The drawing under review shows one solid part. Ordinate dimensions are in mm from its lowest x, y, z. A direction names the side the tool comes from. Coordinates: 2 decimals unless noted, no trailing zeros. Write each loop counter-clockwise with the first axis right and the second up, starting at its lowest first coordinate (ties: lowest second). Pieces come first, ordered by that corner, then holes.
1) Add section B-B, the plane x = 19.25. State the section outline as (y, z) points, then the cut area to 3 significant figures.
2) Mouldability with a two-part tool opening along X and no side actions: class the marked faces 4, 5 and 6 as released by +X, released by -X, zero draft, split by the parting line, or undercut.
3) For line 1 (X direction, y = 27.5, z = 17.5); line 2 (X direction, y = 28, z = 25.5); line 3 (X direction, y = 15.5, z = 16), list the stretches that pass through material, from the lowest coordinate up.
4) Machinability: for the marked faces 1, 2 and 3, which of the approach directions +Z, -Z, +X, -X, +Y, -Y give a long, thin tool a straight path to every point of the face, cutting with its end or side? Answer none if there is none.
5) Add section C-C, the plane x = 11. State the section outline as (y, z) points.
6) For P1, Ø1, axis at x = 16.5, z = 29.5, coming from the +Y side; P2, Ø5, axis at y = 29, z = 10.5, coming from the +X side; P3, Ø10, axis at y = 18, z = 36, coming from the +X side, all flat-tipped, find the tip position at first contact; note any pin that passes through.
7) Add section A-A, the plane z = 21. State the section outline as (x, y) points.
8) Add section D-D, the plane y = 30. State the section outline as (x, z) points.
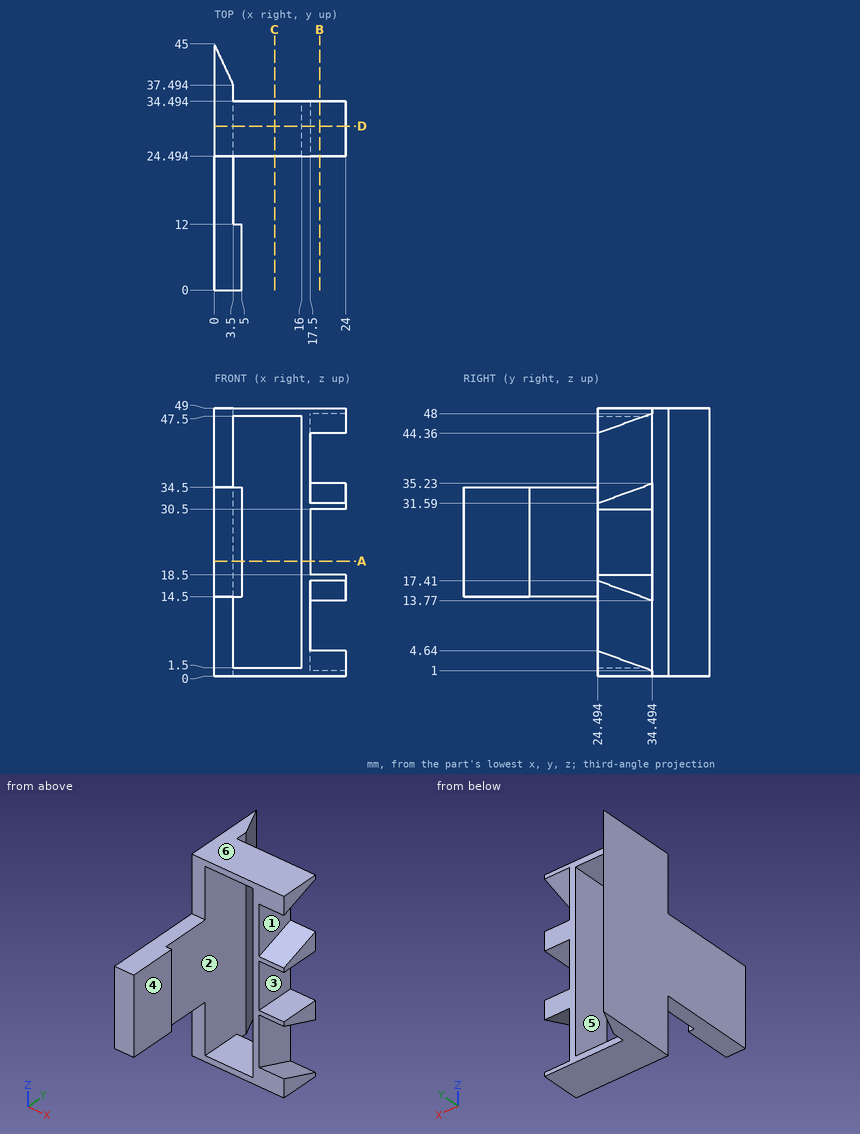
Geometry results:
1. outline: (24.49, 0) - (34.49, 0) - (34.49, 1) - (24.49, 4.64) - close; (24.49, 17.41) - (34.49, 13.77) - (34.49, 18.5) - (24.49, 18.5) - close; (24.49, 30.5) - (34.49, 30.5) - (34.49, 35.23) - (24.49, 31.59) - close; (24.49, 44.36) - (34.49, 48) - (34.49, 49) - (24.49, 49) - close
1. area: 115 mm2
2. face 4: released by +X
2. face 5: undercut
2. face 6: zero draft
3. line 1: x = 0 to 3.5, 16 to 24
3. line 2: x = 0 to 3.5, 16 to 17.5
3. line 3: x = 0 to 3.5
4. face 1: +X
4. face 2: +Y
4. face 3: +X, +Y, -Y
5. outline: (24.49, 0) - (34.49, 0) - (34.49, 1.5) - (24.49, 1.5) - close; (24.49, 47.5) - (34.49, 47.5) - (34.49, 49) - (24.49, 49) - close
6. P1: stops at y = 34.49
6. P2: stops at x = 17.5
6. P3: stops at x = 3.5
7. outline: (0, 0) - (5, 0) - (5, 12) - (3.5, 12) - (3.5, 37.49) - (0, 45) - close; (16, 24.49) - (17.5, 24.49) - (17.5, 34.49) - (16, 34.49) - close
8. outline: (0, 0) - (24, 0) - (24, 2.64) - (17.5, 2.64) - (17.5, 15.41) - (24, 15.41) - (24, 18.5) - (17.5, 18.5) - (17.5, 30.5) - (24, 30.5) - (24, 33.59) - (17.5, 33.59) - (17.5, 46.36) - (24, 46.36) - (24, 49) - (0, 49) - close; hole (3.5, 1.5) - (16, 1.5) - (16, 47.5) - (3.5, 47.5) - close
